Verification items for the finished model (mm, model axes). Round coordinates to 2 decimals unless told otherwise and drop trailing zeros. Order: outer loops, then holes, each group sorted by start corner. A loop starts at its lowest first (then second) coordinate and runs counter-clockwise, first axis right, second up. Notation, with made-up numbers: (-29, 28.25) -> (-20, 28.25) arc R19 ccw to (-20, 57.25) -> close; hole circle Ø8 at (84.5, 63.25). An arc over 180 degrees is marked (long way). Put each result on its own line as item: value.
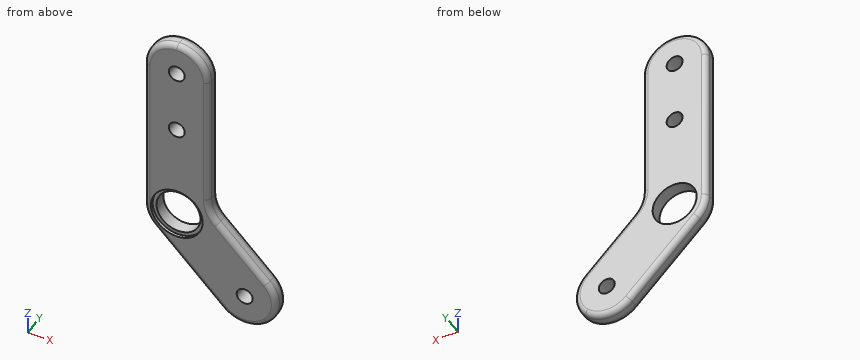
```python
from build123d import *

# Parameters (mm, degrees)
SKETCH1_R           = 3.175
SKETCH1_R_2         = 12.7
SKETCH1_R_3         = 8.73125
BOSS_EXTRUDE1_DEPTH = 6.35
FILLET2_R           = 12.7
FILLET3_R           = 2.116666667
SKETCH3_R           = 10.2489
CUT_EXTRUDE1_DEPTH  = 1.27


with BuildPart() as part:
    # Sketch1 → Boss-Extrude1 (new body)
    # profile 1 of 4: a face of its own
    with BuildSketch(Plane(origin=(0, 0, 0), x_dir=(1, 0, 0), z_dir=(0, 1, 0))):
        with BuildLine():
            Line((-12.7, 31.75), (-12.7, -44.45))
            Line((-12.7, -44.45), (12.7, -44.45))
            Line((12.7, -44.45), (12.7, 26.489487758))
            Line((12.7, 26.489487758), (8.980256121, 22.769743879))
            ThreePointArc((8.980256121, 22.769743879), (-4.860079591, 20.016729937), (-12.7, 31.75))
        make_face()
        with Locations(Location((0, -31.75, 0), (0, 0, 270))):
            Circle(SKETCH1_R, mode=Mode.SUBTRACT)
        with Locations(Location((0, -6.35, 0), (0, 0, 270))):
            Circle(SKETCH1_R, mode=Mode.SUBTRACT)
    # profile 2 of 4: a face of its own
    with BuildSketch(Plane(origin=(0, 0, 0), x_dir=(1, 0, 0), z_dir=(0, 1, 0))):
        with Locations((0, 31.75)):
            Circle(SKETCH1_R_2)
        with Locations(Location((0, 31.75, 0), (0, 0, 270))):
            Circle(SKETCH1_R_3, mode=Mode.SUBTRACT)
    # profile 3 of 4: a face of its own
    with BuildSketch(Plane(origin=(0, 0, 0), x_dir=(1, 0, 0), z_dir=(0, 1, 0))):
        with BuildLine():
            Line((12.7, 31.75), (12.7, 26.489487758))
            Line((12.7, 26.489487758), (44.901280605, 58.690768363))
            Line((44.901280605, 58.690768363), (26.940768363, 76.651280605))
            Line((26.940768363, 76.651280605), (-8.980256121, 40.730256121))
            ThreePointArc((-8.980256121, 40.730256121), (4.860079591, 43.483270063), (12.7, 31.75))
        make_face()
        with Locations(Location((26.940768363, 58.690768363, 0), (0, 0, 270))):
            Circle(SKETCH1_R, mode=Mode.SUBTRACT)
    # profile 4 of 4: a face of its own
    with BuildSketch(Plane(origin=(0, 0, 0), x_dir=(1, 0, 0), z_dir=(0, 1, 0))):
        with BuildLine():
            Line((8.980256121, 22.769743879), (12.7, 26.489487758))
            Line((12.7, 26.489487758), (12.7, 31.75))
            ThreePointArc((12.7, 31.75), (11.733270063, 26.889920409), (8.980256121, 22.769743879))
        make_face()
    extrude(amount=BOSS_EXTRUDE1_DEPTH)

    # Fillet2
    fillet2_edges = [part.edges().sort_by_distance(p)[0] for p in [
        (12.7, 3.175, -26.489487758),
        (26.940768363, 3.175, -76.651280605),
        (44.901280605, 3.175, -58.690768363),
        (-12.7, 3.175, 44.45),
        (12.7, 3.175, 44.45),
    ]]
    fillet(fillet2_edges, radius=FILLET2_R - 0.0001)  # a hair under: the kernel refuses the full size

    # Fillet3
    fillet3_edges = [part.edges().sort_by_distance(p)[0] for p in [
        (-11.733270063, 6.35, -36.610079591),
        (-11.733270063, 0, -36.610079591),
        (26.170404892, 0, -39.95989265),
        (26.170404892, 6.35, -39.95989265),
        (12.7, 0, 5.260541531),
        (12.7, 6.35, 5.260541531),
        (4.490163416, 0, -54.200675658),
        (4.490163416, 6.35, -54.200675658),
        (-12.7, 0, 5e-05),
        (8.98028541, 0, 40.73028541),
        (-8.98028541, 0, 40.73028541),
        (39.640809785, 0, -58.690768363),
        (26.940768363, 0, -71.390809785),
        (-12.7, 6.35, 5e-05),
        (8.98028541, 6.35, 40.73028541),
        (-8.98028541, 6.35, 40.73028541),
        (39.640809785, 6.35, -58.690768363),
        (26.940768363, 6.35, -71.390809785),
        (13.666722325, 0, -26.08905826),
        (13.666722325, 6.35, -26.08905826),
    ]]
    fillet(fillet3_edges, radius=FILLET3_R)

    # Sketch3 → Cut-Extrude1 (cut)
    with BuildSketch(Plane.XZ):
        with Locations(Location((0, -31.75, 0), (0, 0, 270))):
            Circle(SKETCH3_R)
    extrude(amount=-CUT_EXTRUDE1_DEPTH, mode=Mode.SUBTRACT)


solid = part.part
```
Item 1: Material ranges on line 1 along Z through (x, y) = (-0.5, 1); line 2 along X through (y, z) = (2.5, 6.35) (3 decimals); line 3 along X through (y, z) = (2.5, -34), recorded low to high.
Geometry check:
line 1: -48.76 to -41.99, -21.51 to 3.21, 9.49 to 28.61, 34.89 to 44.12
line 2: -12.7 to -3.175, 3.175 to 12.7
line 3: -12.5 to -8.44, 8.44 to 20.21
Item 2: Depth check by flat-ended pin: pin 1 Ø4 at (x, z) = (26.94, -58.69) entering from +Y; pin 2 Ø1.1 at (y, z) = (3, 13) entering from +X; pin 3 Ø1 at (x, y) = (14, 1.5) entering from -Z. Enter the tip coordinate at first touch or a pass-through.
Geometry check:
pin 1: through
pin 2: x = 12.7
pin 3: z = -64.11
Item 3: Sectioned sample at A-A, the plane z = 6.35. Record the boundary of the cut face in (x, y) (3 decimals).
Geometry check:
outline: (-12.7, 2.117) arc R2.117 ccw to (-10.583, 0) -> (-3.175, 0) -> (-3.175, 6.35) -> (-10.583, 6.35) arc R2.117 ccw to (-12.7, 4.233) -> close; (3.175, 0) -> (10.583, 0) arc R2.117 ccw to (12.7, 2.117) -> (12.7, 4.233) arc R2.117 ccw to (10.583, 6.35) -> (3.175, 6.35) -> close
Item 4: Sectioned sample at C-C, the plane z = 22.5. Record the boundary of the cut face in (x, y).
Geometry check:
outline: (-12.7, 2.12) arc R2.12 ccw to (-10.58, 0) -> (10.58, 0) arc R2.12 ccw to (12.7, 2.12) -> (12.7, 4.23) arc R2.12 ccw to (10.58, 6.35) -> (-10.58, 6.35) arc R2.12 ccw to (-12.7, 4.23) -> close
Item 5: Sectioned sample at B-B, the plane y = 5.25. Give the number of separate pieces and of enclosed holes in the cut face, then the cut area to 3 significant figures.
Geometry check:
separate pieces: 1
enclosed holes: 4
area: 2,680 mm2
